from build123d import *

# Parameters (mm, degrees)
F1_DEPTH = 2000
F2_R     = 5
F3_R     = 5
F4_R     = 5
F5_R     = 5


with BuildPart() as f1:
    # F0 (on Front) → F1 (new body)
    with BuildSketch(Plane.XZ):
        Polygon((150, 0), (0, 0), (-150, 0), (-200, 814), (-410, 1069), (-410, 1144), (-560, 1144), (-560, -106), (0, -106), (560, -106), (560, 1144), (410, 1144), (410, 1069), (200, 814), align=None)
    extrude(amount=F1_DEPTH)

    # F2
    f2_edges = [f1.edges().sort_by_distance(p)[0] for p in [
        (-200, -1000, 814),
    ]]
    fillet(f2_edges, radius=F2_R)

    # F3
    f3_edges = [f1.edges().sort_by_distance(p)[0] for p in [
        (-410, -1000, 1069),
    ]]
    fillet(f3_edges, radius=F3_R)

    # F4
    f4_edges = [f1.edges().sort_by_distance(p)[0] for p in [
        (-410, -1000, 1144),
    ]]
    fillet(f4_edges, radius=F4_R)

    # F5
    f5_edges = [f1.edges().sort_by_distance(p)[0] for p in [
        (410, -1000, 1144),
        (200, -1000, 814),
        (150, -1000, 0),
        (410, -1000, 1069),
    ]]
    fillet(f5_edges, radius=F5_R)


solid = f1.part
Model file for the job. Use its own axes, mm. A direction names the side the tool comes from. Round coordinates to 2 decimals unless told otherwise and drop trailing zeros. Loops run counter-clockwise (first coordinate to the right, second up) from the corner with the lowest first, then second, coordinate; pieces in that order, holes last.
1. Band-saw the part on C-C, the plane x = -124. List the corners of the cut face in (y, z), and give its area (3 significant figures).
Check values:
outline: (-2000, -106) - (0, -106) - (0, 0) - (-2000, 0) - close
area: 212,000 mm2
2. Band-saw the part on D-D, the plane z = 781.5. List the corners of the cut face in (x, y).
Check values:
outline: (-560, -2000) - (-198, -2000) - (-198, 0) - (-560, 0) - close; (198, -2000) - (560, -2000) - (560, 0) - (198, 0) - close
3. Mould opens along X. For faces 1 (the flat face through (489, -986, 1144)), 2 (the flat face through (-560, -986, 528)), 3 (the flat face through (0, -986, 0)) say: +X half, -X half, draft (parallel to the pull), parting line (faces both ways), or undercut.
Check values:
face 1: draft
face 2: -X half
face 3: undercut
4. Band-saw the part on A-A, the plane z = 518. List the corners of the cut face in (x, y).
Check values:
outline: (-560, -2000) - (-181.82, -2000) - (-181.82, 0) - (-560, 0) - close; (181.82, -2000) - (560, -2000) - (560, 0) - (181.82, 0) - close
5. Wall check: probe 1 along Z at (x, y) = (-132, -181); probe 2 along X at (y, z) = (-1906, 897.5); probe 3 along X at (y, z) = (-1274.5, 801.5). Give the ranges that are in metal, low to high.
Check values:
probe 1: z = -106 to 0
probe 2: x = -560 to -268.76, 268.76 to 560
probe 3: x = -560 to -199.23, 199.23 to 560
6. Drop a flat-ended pin along its axis: P1, Ø8, axis at x = -61, y = -784.5, coming from the +Z side. Give the stop position or say it passes through.
Check values:
P1: stops at z = 0
7. Tool access for faces 4 (the flat face through (410, -986, 1105)), 5 (the flat face through (-486, -986, 1144)): list every direction of +Z, -Z, +X, -X, +Y, -Y with a clear straight run to the whole face (end or side of a thin tool).
Check values:
face 4: +Z, +Y, -Y
face 5: +Z, +X, -X, +Y, -Y
8. Band-saw the part on B-B, the plane y = -1220. List the corners of the cut face in (x, z), and give its area (3 significant figures).
Check values:
outline: (-560, -106) - (560, -106) - (560, 1144) - (415, 1144) arc R5 ccw to (410, 1139) - (410, 1070.79) arc R5 cw to (408.86, 1067.62) - (201.03, 815.25) arc R5 ccw to (199.9, 812.38) - (150.29, 4.69) arc R5 cw to (145.3, 0) - (-150, 0) - (-199.9, 812.38) arc R5 ccw to (-201.03, 815.25) - (-408.86, 1067.62) arc R5 cw to (-410, 1070.79) - (-410, 1139) arc R5 ccw to (-415, 1144) - (-560, 1144) - close
area: 898,000 mm2
